Source: CAD feature listing. Evaluate the final solid. Frame: model axes, mm. Round coordinates to 2 decimals unless told otherwise and drop trailing zeros. Order: outer loops, then holes, each group sorted by start corner. A loop starts at its lowest first (then second) coordinate and runs counter-clockwise, first axis right, second up. Notation, with made-up numbers: (74, 11) - (123, 11) arc R18 cw to (123, 20) - close; hole circle Ø6 at (88, -14.75). An arc over 180 degrees is marked (long way). Put each result on its own line as item: value. Start each with the question number.
1) Section B-B on x = 10.16. Output: boundary loops of the cut face in (y, z).
2) Line query: probe 1 along Z at (x, y) = (207, -1.35); probe 2 along Z at (x, y) = (10.16, -0.4); probe 3 along Y at (x, z) = (106.5, -79). Output: solid intervals per line, ascending. Write a range as [from, to].
3) Section A-A on x = 107.95. Output: boundary loops of the cut face in (y, z) (3 decimals), then the cut area to 3 significant figures.
4) Contact query for flat-ended pins moving along their axis: P1, Ø4, axis at x = 165, z = -63, coming from the +Y side; P2, Ø2.5, axis at x = 107.95, z = -9.525, coming from the +Y side. Output: stop coordinate, or through.
```python
from build123d import *

# Parameters (mm, degrees)
F1_DEPTH = 1.524
F3_D     = 4.318
F4_R     = 2.159
F5_DEPTH = 0.0254


with BuildPart() as f1:
    # F0 (on Front) → F1 (new body)
    with BuildSketch(Plane.XZ):
        with BuildLine():
            Line((203.2, 0), (12.7, 0))
            ThreePointArc((12.7, 0), (3.7197438789, -3.7197438789), (0, -12.7))
            Line((0, -12.7), (0, -101.6))
            ThreePointArc((0, -101.6), (3.7197438789, -110.5802561211), (12.7, -114.3))
            Line((12.7, -114.3), (203.2, -114.3))
            ThreePointArc((203.2, -114.3), (212.1802561211, -110.5802561211), (215.9, -101.6))
            Line((215.9, -101.6), (215.9, -12.7))
            ThreePointArc((215.9, -12.7), (212.1802561211, -3.7197438789), (203.2, 0))
        make_face()
    extrude(amount=F1_DEPTH)

    # F3 (through all)
    with Locations(Plane.XZ.offset(1.524)):
        with Locations((10.16, -9.525), (107.95, -9.525), (205.74, -9.525), (205.74, -104.775), (107.95, -104.775), (10.16, -104.775)):
            Hole(F3_D / 2)

    # F4 (on face) → F5 (join)
    with BuildSketch(Plane(origin=(0, 0, 0), x_dir=(-1, 0, 0), z_dir=(0, 1, 0))):
        with BuildLine():
            Line((0, -101.6), (0, -12.7))
            ThreePointArc((0, -12.7), (-3.7197438789, -3.7197438789), (-12.7, 0))
            Line((-12.7, 0), (-203.2, 0))
            ThreePointArc((-203.2, 0), (-212.1802561211, -3.7197438789), (-215.9, -12.7))
            Line((-215.9, -12.7), (-215.9, -101.6))
            ThreePointArc((-215.9, -101.6), (-212.1802561211, -110.5802561211), (-203.2, -114.3))
            Line((-203.2, -114.3), (-12.7, -114.3))
            ThreePointArc((-12.7, -114.3), (-3.7197438789, -110.5802561211), (0, -101.6))
        make_face()
        with Locations((-205.74, -104.775)):
            Circle(F4_R, mode=Mode.SUBTRACT)
        with Locations((-107.95, -104.775)):
            Circle(F4_R, mode=Mode.SUBTRACT)
        with Locations((-10.16, -104.775)):
            Circle(F4_R, mode=Mode.SUBTRACT)
        with BuildLine():
            Line((-182.626, -22.225), (-33.274, -22.225))
            ThreePointArc((-33.274, -22.225), (-26.8082155928, -24.9032155928), (-24.13, -31.369))
            Line((-24.13, -31.369), (-24.13, -82.931))
            ThreePointArc((-24.13, -82.931), (-26.8082155928, -89.3967844072), (-33.274, -92.075))
            Line((-33.274, -92.075), (-182.626, -92.075))
            ThreePointArc((-182.626, -92.075), (-189.0917844072, -89.3967844072), (-191.77, -82.931))
            Line((-191.77, -82.931), (-191.77, -31.369))
            ThreePointArc((-191.77, -31.369), (-189.0917844072, -24.9032155928), (-182.626, -22.225))
        make_face(mode=Mode.SUBTRACT)
        with Locations((-205.74, -9.525)):
            Circle(F4_R, mode=Mode.SUBTRACT)
        with Locations((-107.95, -9.525)):
            Circle(F4_R, mode=Mode.SUBTRACT)
        with Locations((-10.16, -9.525)):
            Circle(F4_R, mode=Mode.SUBTRACT)
    extrude(amount=F5_DEPTH)


solid = f1.part
```
Answer sheet:
1. outline: (-1.52, -114.04) - (0.03, -114.04) - (0.03, -106.93) - (-1.52, -106.93) - close; (-1.52, -102.62) - (0.03, -102.62) - (0.03, -11.68) - (-1.52, -11.68) - close; (-1.52, -7.37) - (0.03, -7.37) - (0.03, -0.26) - (-1.52, -0.26) - close
2. probe 1: [-113.72, -106.53], [-103.02, -11.28], [-7.77, -0.58]
2. probe 2: [-114.04, -106.93], [-102.62, -11.68], [-7.37, -0.26]
2. probe 3: [-1.52, 0]
3. outline: (-1.524, -114.3) - (0.025, -114.3) - (0.025, -106.934) - (-1.524, -106.934) - close; (-1.524, -102.616) - (0.025, -102.616) - (0.025, -92.075) - (0, -92.075) - (0, -22.225) - (0.025, -22.225) - (0.025, -11.684) - (-1.524, -11.684) - close; (-1.524, -7.366) - (0.025, -7.366) - (0.025, 0) - (-1.524, 0) - close
3. area: 162 mm^2
4. P1: y = 0
4. P2: through
